Verification items for the finished model (mm, model axes). A direction names the side the tool comes from. Coordinates: 2 decimals unless noted, no trailing zeros. Write each loop counter-clockwise with the first axis right and the second up, starting at its lowest first coordinate (ties: lowest second). Pieces come first, ordered by that corner, then holes. Notation, with made-up numbers: (85.25, 12) -> (130.25, 12) arc R24 cw to (130.25, 31) -> close; hole circle Ø3 at (6, 24.5). An arc over 180 degrees is marked (long way). Write each question's results on one line, items separated by ' | '. Start each with the question number.
Autodesk Inventor part; units mm, degrees
ref_plane "YZ Plane" through (0, 0, 0) normal (1, 0, 0) x (0, 1, 0)
ref_plane "XZ Plane" through (0, 0, 0) normal (0, 1, 0) x (-1, 0, 0)
ref_plane "XY Plane" through (0, 0, 0) normal (0, 0, 1) x (1, 0, 0)
sketch "Sketch1" plane through (0, 0, 0) normal (0, 1, 0) x (-1, 0, 0)
  line L0 (-0.75, -1.6) -> (0.75, -1.6)
  line L1 (0.75, -1.6) -> (0.75, 1.6)
  line L2 (0.75, 1.6) -> (-0.75, 1.6)
  line L3 (-0.75, 1.6) -> (-0.75, -1.6)
  line L4 (-0.75, -1.6) -> (0.75, 1.6) construction
  line L5 (0.75, -1.6) -> (-0.75, 1.6) construction
  line L6 (0.75, 1.6) -> (-0.75, 1.6)
  line L7 (-0.75, 1.6) -> (-0.75, 2.6)
  line L8 (-0.75, 2.6) -> (0.75, 2.6)
  line L9 (0.75, 2.6) -> (0.75, 1.6)
  line L10 (-0.75, -1.6) -> (0.75, -1.6)
  line L11 (0.75, -1.6) -> (0.75, -2.6)
  line L12 (0.75, -2.6) -> (-0.75, -2.6)
  line L13 (-0.75, -2.6) -> (-0.75, -1.6)
  point P0 (0, 0)
  point P1 (0.75, -1.6)
  dimension "d0" = 3.2
  dimension "d1" = 1.5
  dimension "d2" = 1
  dimension "d3" = 1
extrude "Extrusion1" add sketch "Sketch1" along normal blind 0.5 contours L0 L11 L12 L13 | L7 L8 L9 L2
sketch "Sketch2" plane through (0.75, 0, 2.6) normal (1, 0, 0) x (0, 0, -1)
  line L0 (0, 0.5) -> (1, 0.5)
  line L1 (0.85, 0.5) -> (4.35, 0.5)
  line L2 (4.35, 0.5) -> (4.35, 1.5)
  line L3 (4.35, 1.5) -> (0.85, 1.5)
  line L4 (0.85, 1.5) -> (0.85, 0.5)
  line L5 (0.85, 1.5) -> (0, 0.5)
  line L6 (5.2, 0) -> (5.2, 0.5)
  line L7 (4.35, 1.5) -> (5.2, 0.5)
  line L8 (0, 0) -> (1, 0) construction
  line L9 (0, 0) -> (5.2, 0) construction
  line L10 (2.6, 0) -> (2.6, 2.5684) construction
  line L11 (0, 0.5) -> (5.2, 0.5)
  point P0 (2.6, 0.5)
  dimension "d10" = 3.5
  dimension "d19" = 1
extrude "Extrusion3" add sketch "Sketch2" against normal blind 1.5
sketch "Sketch5" plane through (0.75, 1.5, 1.75) normal (0, 1, 0) x (1, 0, 0)
  line L0 (-1.5, 0) -> (-1.5, 3.5)
  line L1 (0, 3.5) -> (0, 0)
  line L2 (-1.5, 3.5) -> (0, 3.5)
  line L3 (0, 3.5) -> (0, 0)
  line L4 (0, 0) -> (-1.5, 0)
  line L5 (-1.5, 0) -> (-1.5, 3.5)
  point P0 (-0.75, 1.75)
  point P1 (0, 3.5)
  point P2 (-1.5, 0)
extrude "Extrusion5" add sketch "Sketch5" along normal blind 2
sketch "Sketch6" plane through (0.75, 3.5, 1.75) normal (0, 1, 0) x (1, 0, 0)
  line L0 (-1.5, 3) -> (0, 3)
  line L1 (0, 3) -> (0, 0.5)
  line L2 (0, 0.5) -> (-1.5, 0.5)
  line L3 (-1.5, 0.5) -> (-1.5, 3)
  line L4 (0, 0) -> (0, 3.5) construction
  line L5 (0, 0) -> (0, 0.5) construction
  line L6 (-0.75, 3) -> (-0.75, 3.5) construction
  line L7 (0, 3.5) -> (-1.5, 3.5) construction
  line L8 (-0.75, 0.5) -> (-0.75, 0) construction
  point P0 (-0.75, 1.75)
  point P1 (-1.5, 1.75)
  point P2 (0, 1.75)
  dimension "d20" = 2.5
extrude "Extrusion6" add sketch "Sketch6" along normal blind 5.5
fillet "Fillet1" radius 0.6 4 edges at (0, 9, -1.25) (-0.75, 9, 0) (0, 9, 1.25) (0.75, 9, 0)
sketch "Sketch7" plane through (0, 0, 0) normal (0, -1, 0) x (1, 0, 0)
  line L0 (-0.75, 2.6) -> (0.75, 2.6)
  line L1 (-0.75, -2.6) -> (0.75, -2.6)
  line L2 (0.75, -2.6) -> (0.75, 2.6)
  line L3 (0.75, 2.6) -> (-0.75, 2.6)
  line L4 (-0.75, 2.6) -> (-0.75, -2.6)
  line L5 (-0.75, -2.6) -> (0.75, 2.6) construction
  line L6 (0.75, -2.6) -> (-0.75, 2.6) construction
  point P0 (0, 0)
extrude "Extrusion7" cut sketch "Sketch7" against normal blind 0.5
sketch "Sketch8" plane through (0.75, 0.5, -2.6) normal (0, -1, 0) x (1, 0, 0)
  line L0 (-1.5, 5.2) -> (0, 5.2)
  line L1 (0, 4.35) -> (-1.5, 4.35)
  line L2 (0, 5.2) -> (-1.5, 5.2)
  line L3 (-1.5, 5.2) -> (-1.5, 4.35)
  line L4 (-1.5, 4.35) -> (0, 4.35)
  line L5 (0, 4.35) -> (0, 5.2)
  line L6 (0, 0) -> (-1.5, 0)
  line L7 (0, 0.85) -> (-1.5, 0.85)
  line L8 (0, 0) -> (-1.5, 0)
  line L9 (-1.5, 0) -> (-1.5, 0.85)
  line L10 (-1.5, 0.85) -> (0, 0.85)
  line L11 (0, 0.85) -> (0, 0)
  point P0 (-0.75, 2.6)
  point P1 (0, 0.85)
extrude "Extrusion8" cut sketch "Sketch8" against normal blind 2
sketch "Sketch4" plane through (0.75, 1.5, 1.75) normal (0, 1, 0) x (1, 0, 0)
  line L0 (-1.5, 3) -> (0, 3)
  line L1 (0, 3) -> (0, 0.5)
  line L2 (0, 0.5) -> (-1.5, 0.5)
  line L3 (-1.5, 0.5) -> (-1.5, 3)
  line L4 (-1.5, 0) -> (-1.5, 3.5)
  line L5 (0, 3.5) -> (0, 0)
  line L6 (0, 3.5) -> (-1.5, 3.5)
  point P0 (-0.75, 1.75)
  point P1 (-1.5, 1.75)
  point P2 (0, 1.75)
  point P3 (-0.75, 3)
  dimension "d13" = 2.5
  dimension "d14" = 0.5
properties part number "LightPipeThin"
1. Sectioned sample at B-B on y = 3.75. Record the cut outline in (x, z), plus the area to 3 significant figures.
2. Sectioned sample at C-C on z = 1.5. Record the cut outline in (x, y).
3. Tool access check on faces 1 (the flat face through (0.75, 4, 0)), 2 (the flat face through (0, 6, -1.25)), 3 (the flat face through (0, 6, 1.25)). Record the directions out of +Z, -Z, +X, -X, +Y, -Y that give a thin tool (end or side, any length) a straight path to the whole face; none if there is none.
4. Depth check by flat-ended pin: pin 1 Ø0.8 at (x, y) = (0, 5) entering from +Z. Enter the tip coordinate at first touch or a pass-through.
5. Sectioned sample at A-A on x = 0.55. Record the cut outline in (y, z), plus the area to 3 significant figures.
6. Sectioned sample at D-D on x = -0.4. Record the cut outline in (y, z), plus the area to 3 significant figures.
7. Material ranges on probe 1 along Z at (x, y) = (0.25, 5.25); probe 2 along Y at (x, z) = (-0.3, -1.5); probe 3 along Y at (x, z) = (0.3, 0.75), recorded low to high. Write a range as from..to.
Computed values:
1) outline: (-0.75, -1.25) -> (0.75, -1.25) -> (0.75, 1.25) -> (-0.75, 1.25) -> close | area: 3.75 mm^2
2) outline: (-0.75, 0.5) -> (0.75, 0.5) -> (0.75, 3.5) -> (-0.75, 3.5) -> close
3) face 1: +Z, -Z, +X, +Y, -Y | face 2: -Z, +X, -X, +Y | face 3: +Z, +X, -X, +Y
4) pin 1: stops at z = 1.25
5) outline: (0.5, -1.75) -> (3.5, -1.75) -> (3.5, -1.25) -> (8.4, -1.25) arc R0.6 ccw to (8.85, -1.05) -> (8.85, 1.05) arc R0.6 ccw to (8.4, 1.25) -> (3.5, 1.25) -> (3.5, 1.75) -> (0.5, 1.75) -> close | area: 23.8 mm^2
6) outline: (0.5, -1.75) -> (3.5, -1.75) -> (3.5, -1.25) -> (8.4, -1.25) arc R0.6 ccw to (8.95, -0.9) -> (8.95, 0.9) arc R0.6 ccw to (8.4, 1.25) -> (3.5, 1.25) -> (3.5, 1.75) -> (0.5, 1.75) -> close | area: 24.0 mm^2
7) probe 1: z = -1.25..1.25 | probe 2: y = 0.5..3.5 | probe 3: y = 0.5..8.98
